Verification items for this drawing (mm, ordinates from the low corner). A direction names the side the tool comes from. Give positions to 0.01 mm unless a question says otherwise; leave off trailing zeros. Write each loop counter-clockwise with the first axis right and the second up, starting at its lowest first coordinate (ties: lowest second). Pieces come first, ordered by that corner, then holes. Notation, with made-up numbers: (-29.5, 72.25) -> (17.5, 72.25) arc R21 ccw to (17.5, 98.25) -> close; hole circle Ø3 at (-9, -24). An arc over 180 degrees is marked (long way). Use one line per item in the form item = value. Start each with the question number.
(1) Scan lines: L1, parallel to Z at x = 4.25, y = 1.25; L2, parallel to X at y = 3.5, z = 11.25; L3, parallel to Y at x = 6.75, z = 5.25. Record each from-to range of solid material in increasing order.
(2) Section check C-C, the plane z = 5.5. Record the cut outline in (x, y), plus the area to 3 significant figures.
(3) Section check A-A, the plane x = 3.6. Record the cut outline in (y, z).
(4) Set-up check for the marked faces 1, 2 and 3: record each of +Z, -Z, +X, -X, +Y, -Y from which the full face is reachable in a straight line by a thin tool's end or side.
(5) Section check D-D, the plane z = 2. Record the cut outline in (x, y), plus the area to 3 significant figures.
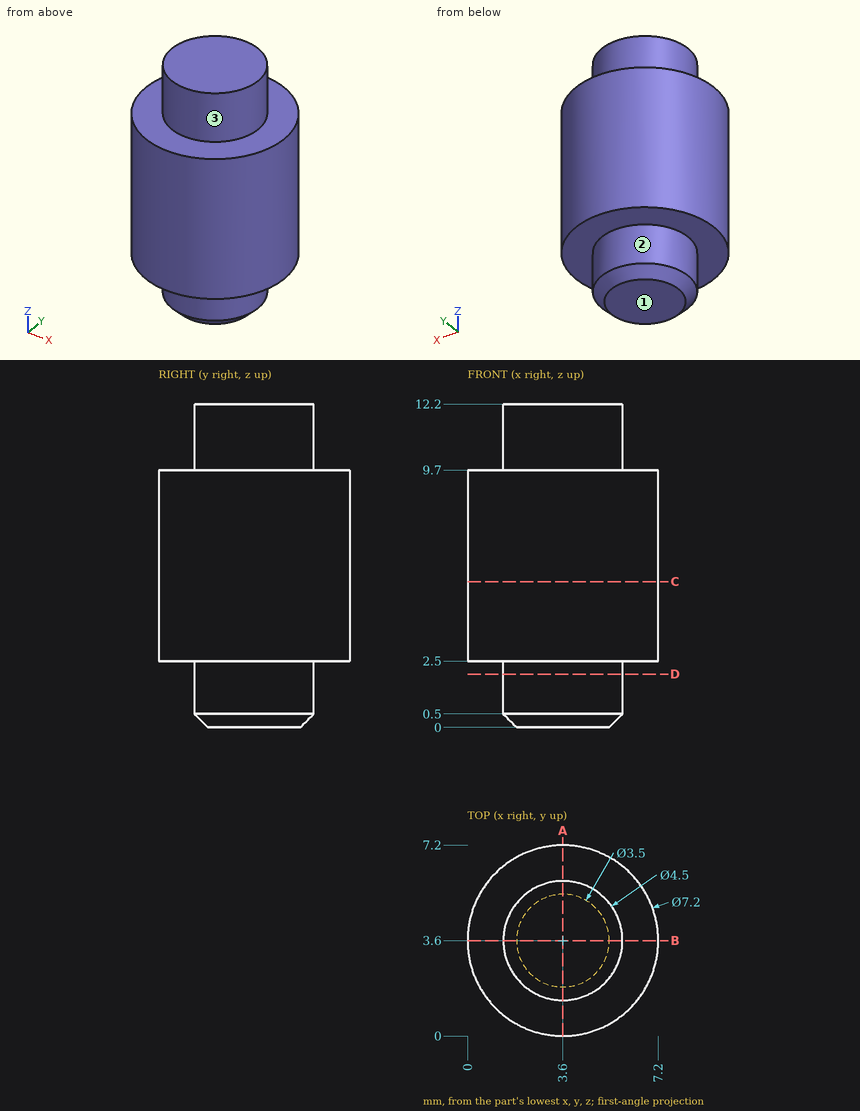
Completed:
q1.L1 = 2.5 to 9.7
q1.L2 = 1.35 to 5.85
q1.L3 = 1.86 to 5.34
q2.outline = circle Ø7.2 at (3.6, 3.6)
q2.area = 40.7 mm²
q3.outline = (0, 2.5) -> (1.35, 2.5) -> (1.35, 0.5) -> (1.85, 0) -> (5.35, 0) -> (5.85, 0.5) -> (5.85, 2.5) -> (7.2, 2.5) -> (7.2, 9.7) -> (5.85, 9.7) -> (5.85, 12.2) -> (1.35, 12.2) -> (1.35, 9.7) -> (0, 9.7) -> close
q4.face_1 = -Z, +X, -X, +Y, -Y
q4.face_2 = -Z
q4.face_3 = +Z
q5.outline = circle Ø4.5 at (3.6, 3.6)
q5.area = 15.9 mm²
